from build123d import *

# Parameters (mm, degrees)
EXTRUDE_1_DEPTH     = 4.6
SKETCH_1_R          = 2.625
SKETCH_1_W          = 40.4
SKETCH_1_H          = 4.6
CUT_EXTRUDE_1_DEPTH = 4.6
FILLET_2_R          = 4
FILLET_3_R          = 9.2625


with BuildPart() as part:
    # 草图3 → 凸台-拉伸1 (new body)
    with BuildSketch(Plane(origin=(0, 0, 0), x_dir=(1, 0, 0), z_dir=(0, 1, 0))):
        Polygon((-18.5, -28), (40, -28), (40, 28), (-18.5, 28), (-18.5, 36), (-45, 36), (-45, 28), (-45, -28), (-45, -36), (-18.5, -36), align=None)
    extrude(amount=EXTRUDE_1_DEPTH)

    # 草图1 → 切除-拉伸1 (cut)
    with BuildSketch(Plane(origin=(0, 0, 0), x_dir=(1, 0, 0), z_dir=(0, 1, 0))):
        with Locations(Location((-31.75, 20.6375, 0), (0, 0, 90))):
            Circle(SKETCH_1_R)
        with Locations(Location((31.75, 20.6375, 0), (0, 0, 90))):
            Circle(SKETCH_1_R)
        with Locations(Location((31.75, -20.6375, 0), (0, 0, 90))):
            Circle(SKETCH_1_R)
        with Locations(Location((-31.75, -20.6375, 0), (0, 0, 90))):
            Circle(SKETCH_1_R)
        with Locations((-13, -10.4375)):
            Rectangle(SKETCH_1_W, SKETCH_1_H)
        with Locations((-13, 10.4375)):
            Rectangle(SKETCH_1_W, SKETCH_1_H)
        Polygon((-3.25, -26.5375), (-3.25, -14.7375), (18.75, -14.7375), (18.75, -26.5375), (18.75, -29.869530405), (-3.25, -29.869530405), align=None)
        Polygon((-3.25, 14.7375), (18.75, 14.7375), (18.75, 26.5375), (18.75, 29.869530405), (-3.25, 29.869530405), (-3.25, 26.5375), align=None)
    extrude(amount=CUT_EXTRUDE_1_DEPTH, mode=Mode.SUBTRACT)

    # 圆角2
    fillet_2_edges = [part.edges().sort_by_distance(p)[0] for p in [
        (-3.25, 2.3, -28),
        (18.75, 2.3, -28),
        (40, 2.3, -28),
        (40, 2.3, 28),
        (18.75, 2.3, 28),
        (-3.25, 2.3, 28),
        (18.75, 2.3, -14.7375),
        (18.75, 2.3, 14.7375),
        (-18.5, 2.3, 28),
        (-18.5, 2.3, 36),
        (-45, 2.3, 36),
        (-45, 2.3, -36),
        (-18.5, 2.3, -36),
        (-18.5, 2.3, -28),
    ]]
    fillet(fillet_2_edges, radius=FILLET_2_R - 0.0001)  # a hair under: the kernel refuses the full size

    # 圆角3
    fillet_3_edges = [part.edges().sort_by_distance(p)[0] for p in [
        (-3.25, 2.3, -14.7375),
        (-3.25, 2.3, 14.7375),
    ]]
    fillet(fillet_3_edges, radius=FILLET_3_R)


solid = part.part
Input: part model. Units: mm. Frame: model coordinates. A direction names the side the tool comes from. Round coordinates to 2 decimals unless told otherwise and drop trailing zeros. Write each loop counter-clockwise with the first axis right and the second up, starting at its lowest first coordinate (ties: lowest second). Pieces come first, ordered by that corner, then holes.
1) Cut plane B-B (x = 31.75). Return the cut outline in (y, z).
2) Draft query along X for faces 1 (the flat face through (40, 2, 0)), 2 (the flat face through (10, 2, -14.738)), 3 (the flat face through (-11, 2, 28)). Return one class per face: pulls with the +X half, pulls with the -X half, needs draft (parallel to the pull), parting line crosses it, or undercut.
3) Reachability of faces 4 (the cylindrical face through (-4.453, 2.332, -26.859)), 5 (the flat face through (-33.2, 2, -10)), 6 (the cylindrical face through (-4.453, 2.268, 26.859)), 7 (the flat face through (29, 2, 28)) from +Z, -Z, +X, -X, +Y, -Y: full face, straight path, thin tool, end or side. Return the list, or none.
4) Contact query for flat-ended pins moving along their axis: P1, Ø3, axis at x = -31.75, z = -20.64, coming from the +Y side; P2, Ø1.5, axis at x = -8, y = 1.5, coming from the -Z side; P3, Ø1.4, axis at x = -6.5, y = 2.5, coming from the +Z side. Output: stop coordinate, or through.
5) Cut plane A-A (x = -31.75). Return the cut outline in (y, z), then the cut area to 3 significant figures.
6) Cut plane C-C (z = 21). Return the cut outline in (x, y).
7) Cut plane D-D (y = 1.65). Count the separate pieces of the cut face and the enclosed holes in it, then the cut area to 3 significant figures.
8) Ray query, L1, parallel to Z at x = -31.75, y = 1.05; L2, parallel to Z at x = 31.75, y = 1.75; L3, parallel to X at y = 0.2, z = 10. Return the intervals inside material, ascending.
Geometry says:
1. outline: (0, -28) - (4.6, -28) - (4.6, -23.26) - (0, -23.26) - close; (0, -18.01) - (4.6, -18.01) - (4.6, 18.01) - (0, 18.01) - close; (0, 23.26) - (4.6, 23.26) - (4.6, 28) - (0, 28) - close
2. face 1: pulls with the +X half
2. face 2: undercut
2. face 3: needs draft
3. face 4: -Z, +Y, -Y
3. face 5: +Y, -Y
3. face 6: +Z, +Y, -Y
3. face 7: +Z, +X, +Y, -Y
4. P1: passes through
4. P2: stops at z = -28
4. P3: stops at z = 28
5. outline: (0, -36) - (4.6, -36) - (4.6, -23.26) - (0, -23.26) - close; (0, -18.01) - (4.6, -18.01) - (4.6, -12.74) - (0, -12.74) - close; (0, -8.14) - (4.6, -8.14) - (4.6, 8.14) - (0, 8.14) - close; (0, 12.74) - (4.6, 12.74) - (4.6, 18.01) - (0, 18.01) - close; (0, 23.26) - (4.6, 23.26) - (4.6, 36) - (0, 36) - close
5. area: 241 mm2
6. outline: (-45, 0) - (-34.35, 0) - (-34.35, 4.6) - (-45, 4.6) - close; (-29.15, 0) - (-2.75, 0) - (-2.75, 4.6) - (-29.15, 4.6) - close; (18.75, 0) - (29.15, 0) - (29.15, 4.6) - (18.75, 4.6) - close; (34.35, 0) - (40, 0) - (40, 4.6) - (34.35, 4.6) - close
7. separate pieces: 1
7. enclosed holes: 6
7. area: 4,160 mm2
8. L1: z = -36 to -23.26, -18.01 to -12.74, -8.14 to 8.14, 12.74 to 18.01, 23.26 to 36
8. L2: z = -28 to -23.26, -18.01 to 18.01, 23.26 to 28
8. L3: x = -45 to -33.2, 7.2 to 40
